Check sheet for the drawn part. Datum: minimum x, y, z corner. Units: mm. A direction names the side the tool comes from. Coordinates: 2 decimals unless noted, no trailing zeros. Loops run counter-clockwise (first coordinate to the right, second up) from the corner with the lowest first, then second, coordinate; pieces in that order, holes last.
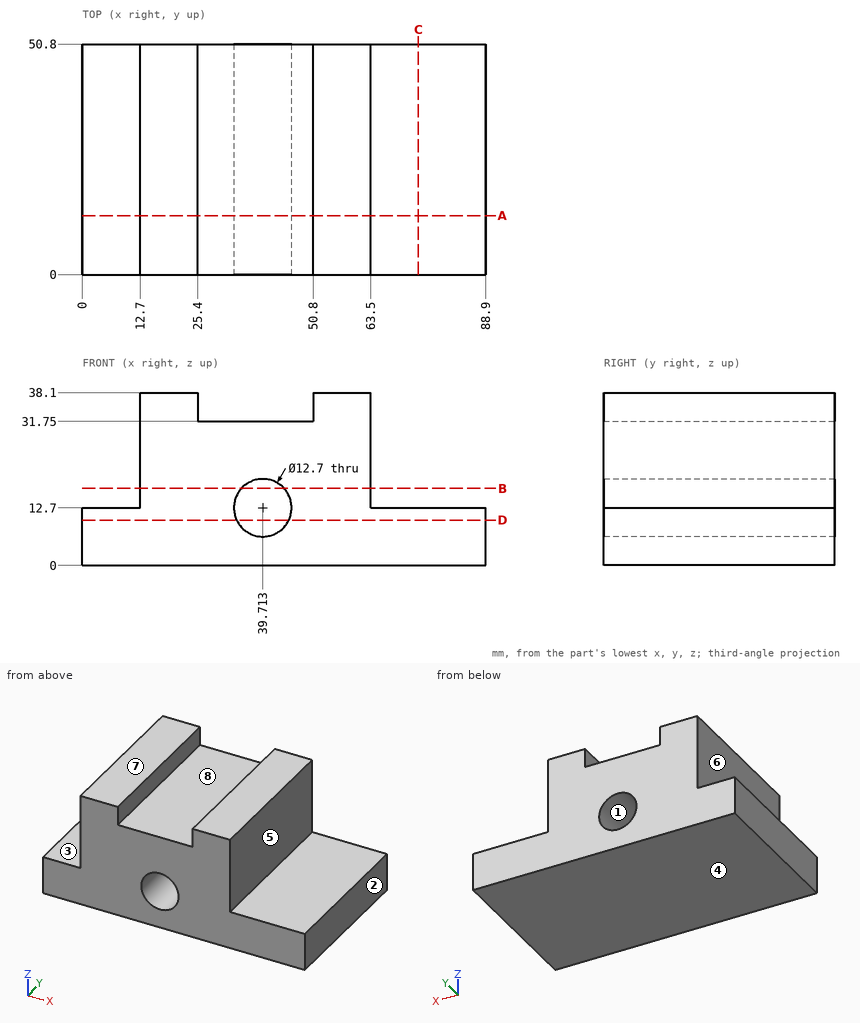
1) Mould release check, pull along Z, two halves, no side actions. Record for the marked faces 1, 2 and 3: +Z half, -Z half, draft (parallel to the pull), parting line (faces both ways), or undercut.
Answer sheet:
face 1: undercut
face 2: draft
face 3: +Z half
2) Depth check by flat-ended pin: pin 1 (1.9 mm diameter, centred on y = 24, z = 34.5, fed in from -X); pin 2 (4 mm diameter, centred on x = 8.5, y = 21.5, fed in from +Z); pin 3 (1 mm diameter, centred on y = 35.5, z = 28.5, fed in from +X). Enter the tip coordinate at first touch or a pass-through.
Answer sheet:
pin 1: stops at x = 12.7
pin 2: stops at z = 12.7
pin 3: stops at x = 63.5
3) Scan lines: line 1 (Z direction, x = 74, y = 48.5); line 2 (X direction, y = 21, z = 22); line 3 (Z direction, x = 43.5, y = 8.5). Record each from-to range of solid material in increasing order.
Answer sheet:
line 1: z = 0 to 12.7
line 2: x = 12.7 to 63.5
line 3: z = 0 to 7.6, 17.8 to 31.75
4) Section check A-A on y = 13. Enter the section's corners in (x, z), plus the area to 3 significant figures.
Answer sheet:
outline: (0, 0) - (88.9, 0) - (88.9, 12.7) - (63.5, 12.7) - (63.5, 38.1) - (50.8, 38.1) - (50.8, 31.75) - (25.4, 31.75) - (25.4, 38.1) - (12.7, 38.1) - (12.7, 12.7) - (0, 12.7) - close; hole circle Ø12.7 at (39.71, 12.7)
area: 2,130 mm2
5) Section check C-C on x = 74. Enter the section's corners in (y, z).
Answer sheet:
outline: (0, 0) - (50.8, 0) - (50.8, 12.7) - (0, 12.7) - close
6) Section check B-B on z = 17. Enter the section's corners in (x, y), plus the area to 3 significant figures.
Answer sheet:
outline: (12.7, 0) - (35.04, 0) - (35.04, 50.8) - (12.7, 50.8) - close; (44.39, 0) - (63.5, 0) - (63.5, 50.8) - (44.39, 50.8) - close
area: 2,110 mm2
7) Section check D-D on z = 10. Enter the section's corners in (x, y), plus the area to 3 significant figures.
Answer sheet:
outline: (0, 0) - (33.97, 0) - (33.97, 50.8) - (0, 50.8) - close; (45.46, 0) - (88.9, 0) - (88.9, 50.8) - (45.46, 50.8) - close
area: 3,930 mm2
8) Set-up check for the marked faces 4, 5, 6, 7 and 8: record each of +Z, -Z, +X, -X, +Y, -Y from which the full face is reachable in a straight line by a thin tool's end or side.
Answer sheet:
face 4: -Z, +X, -X, +Y, -Y
face 5: +Z, +X, +Y, -Y
face 6: +Z, -X, +Y, -Y
face 7: +Z, +X, -X, +Y, -Y
face 8: +Z, +Y, -Y
